```python
from build123d import *

# Parameters (mm, degrees)
F0_W     = 70
F0_H     = 136
F1_DEPTH = 8
F2_R     = 15
F3_R     = 5.08
F4_R     = 1.27


with BuildPart() as f1:
    # F0 (on Front) → F1 (new body)
    with BuildSketch(Plane.XZ):
        Rectangle(F0_W, F0_H)
    extrude(amount=F1_DEPTH)

    # F2
    f2_edges = [f1.edges().sort_by_distance(p)[0] for p in [
        (35, -4, 68),
        (-35, -4, 68),
        (35, -4, -68),
        (-35, -4, -68),
    ]]
    fillet(f2_edges, radius=F2_R)

    # F3
    f3_edges = [f1.edges().sort_by_distance(p)[0] for p in [
        (0, 0, 68),
        (30.606602, 0, 63.606602),
    ]]
    fillet(f3_edges, radius=F3_R)

    # F4
    f4_edges = [f1.edges().sort_by_distance(p)[0] for p in [
        (-30.606602, -8, 63.606602),
        (0, -8, 68),
    ]]
    fillet(f4_edges, radius=F4_R)


solid = f1.part
```
Work out the finished part from the listing and answer in its coordinate system (mm). Coordinates: 2 decimals unless noted, no trailing zeros. Write each loop counter-clockwise with the first axis right and the second up, starting at its lowest first coordinate (ties: lowest second). Pieces come first, ordered by that corner, then holes. Notation, with made-up numbers: (-6.75, 18.25) - (42.25, 18.25) arc R29 ccw to (42.25, 48.25) - close; hole circle Ø7 at (-14.75, 89.5). An arc over 180 degrees is marked (long way). Answer as a JSON object with one key per item and string values.
Q1. Consider L1, parallel to X at y = -1.75, z = -40.5; L2, parallel to X at y = -5, z = -8.5; L3, parallel to Z at x = -2, y = -3.75. Determine where each line is inside the solid, lowest interval first. Write a range as from..to.
Results list:
{"L1": "x = -33.76..33.76", "L2": "x = -35..35", "L3": "z = -67.82..67.82"}
Q2. Find section A-A (z = 18). Write down the section's boundary in (x, y), plus the area to 3 significant figures.
Results list:
{"outline": "(-35, -6.73) arc R1.27 ccw to (-33.73, -8) - (33.73, -8) arc R1.27 ccw to (35, -6.73) - (35, -5.08) arc R5.08 ccw to (29.92, 0) - (-29.92, 0) arc R5.08 ccw to (-35, -5.08) - close", "area": "548 mm^2"}
Q3. Find section B-B (y = -2). Write down the section's boundary in (x, z).
Results list:
{"outline": "(-33.96, -53) arc R13.96 ccw to (-20, -66.96) - (20, -66.96) arc R13.96 ccw to (33.96, -53) - (33.96, 53) arc R13.96 ccw to (20, 66.96) - (-20, 66.96) arc R13.96 ccw to (-33.96, 53) - close"}
Q4. Given pin 1 Ø4 at (x, y) = (2, -2.5) entering from -Z; pin 2 Ø4 at (x, y) = (-1.5, -1) entering from +Z, each flat-ended and moving along its own axis, determine where each tip first touches the part or whether it passes through.
Results list:
{"pin 1": "stops at z = -67.97", "pin 2": "stops at z = 67.55"}
